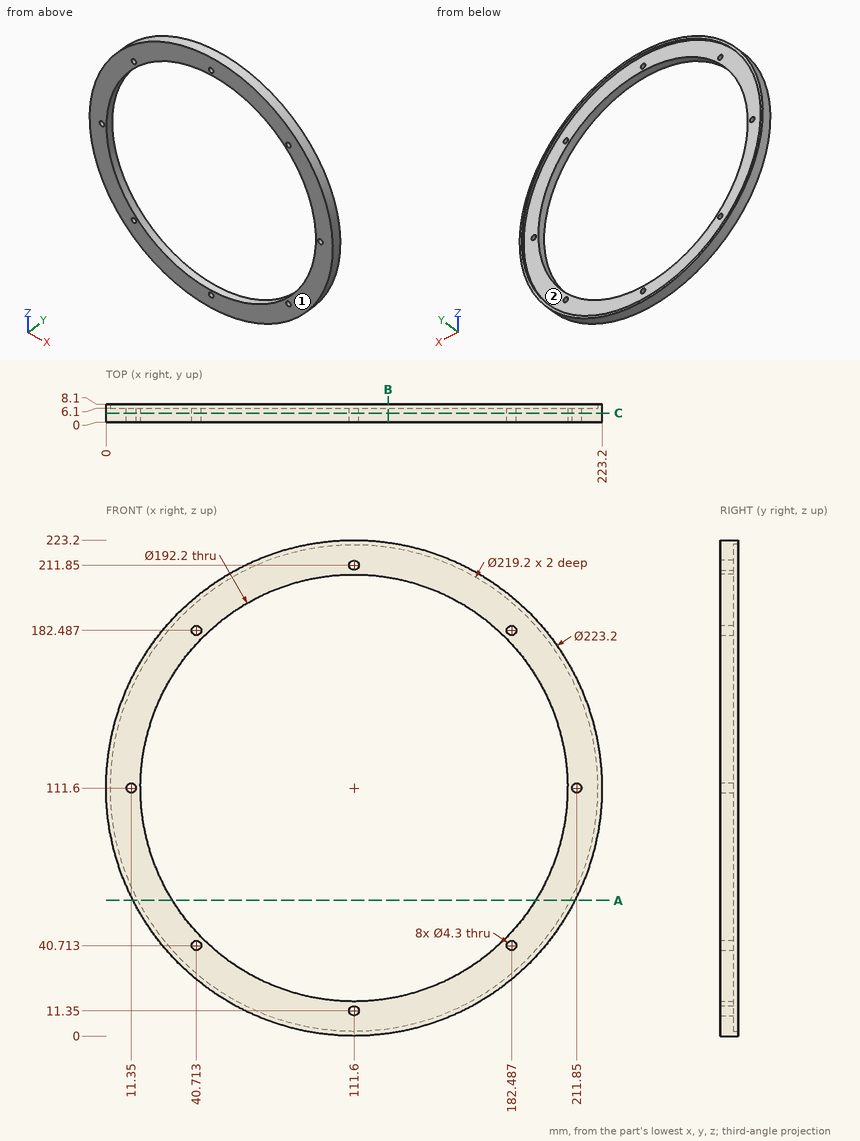
Could you check a few things on this drawing? It's one solid part, dimensions in mm from its lowest x, y, z. Round coordinates to 2 decimals unless told otherwise and drop trailing zeros. Loops run counter-clockwise (first coordinate to the right, second up) from the corner with the lowest first, then second, coordinate; pieces in that order, holes last. Notation, with made-up numbers: (46, 26.25) -> (75, 26.25) arc R12 cw to (75, 41.25) -> close; hole circle Ø2 at (-11.5, 34.25). An arc over 180 degrees is marked (long way). One line per item, written item: value. Start each with the question number.
1. If we section it at B-B, the plane x = 127: Write out the boundary of the cut face in (y, z), then the cut area to 3 significant figures.
2. For pin 1 (3.5 mm diameter, centred on x = 211.85, z = 111.6, fed in from -Y); pin 2 (5 mm diameter, centred on x = 11.35, z = 111.6, fed in from +Y); pin 3 (4 mm diameter, centred on x = 80.5, y = 3, fed in from -Z); pin 4 (1 mm diameter, centred on x = 139.5, y = 6, fed in from +Z), each with a flat end and sliding along its axis, tell me the tip position at first contact or that it passes through.
3. If we section it at C-C, the plane y = 4: Give the number of separate pieces and of enclosed holes in the cut face, then the cut area to 4 significant figures.
4. If we section it at A-A, the plane z = 61: Write out the boundary of the cut face in (x, y).
5. If I drill on probe 1 along X at (y, z) = (4.5, 40) (1 decimal); probe 2 along X at (y, z) = (4, 111.6); probe 3 along Z at (x, y) = (97, 5) (1 decimal), over which ranges is the centre line in solid material (lowest first)?
6. If we mould it in two halves opening along Z, with no side actions, what happens to the marked faces 1 and 2? For each: pulls with the +Z half, pulls with the -Z half, needs draft (parallel to the pull), parting line crosses it, or undercut.
Calculated:
1. outline: (0, 1.07) -> (8.1, 1.07) -> (8.1, 3.09) -> (6.1, 3.09) -> (6.1, 16.74) -> (0, 16.74) -> close; (0, 206.46) -> (6.1, 206.46) -> (6.1, 220.11) -> (8.1, 220.11) -> (8.1, 222.13) -> (0, 222.13) -> close
1. area: 199 mm²
2. pin 1: passes through
2. pin 2: stops at y = 6.1
2. pin 3: stops at z = 3.86
2. pin 4: stops at z = 219.78
3. separate pieces: 1
3. enclosed holes: 9
3. area: 10,000 mm²
4. outline: (12.13, 0) -> (29.9, 0) -> (29.9, 6.1) -> (14.38, 6.1) -> (14.38, 8.1) -> (12.13, 8.1) -> close; (193.3, 0) -> (211.07, 0) -> (211.07, 8.1) -> (208.82, 8.1) -> (208.82, 6.1) -> (193.3, 6.1) -> close
5. probe 1: x = 26 to 38.7, 42.7 to 47.5, 175.7 to 180.5, 184.5 to 197.2
5. probe 2: x = 0 to 9.2, 13.5 to 15.5, 207.7 to 209.7, 214 to 223.2
5. probe 3: z = 1 to 16.6, 206.6 to 222.2
6. face 1: needs draft
6. face 2: undercut
